Can you work these out from the model? Positions are in its coordinate system, mm. Coordinates: 2 decimals unless noted, no trailing zeros. Order: outer loops, then holes, each group sorted by start corner. A loop starts at its lowest first (then second) coordinate and runs counter-clockwise, first axis right, second up. Notation, with made-up numbers: (31, 31) -> (47, 31) arc R29 cw to (47, 61) -> close; hole circle Ø1 at (31, 22). An arc over 180 degrees is marked (long way). Answer as a JSON object with one key per item and string values. Group by question number.
(1) I want a section at D-D, the plane y = -48. List the corners of the cut face in (x, z) for me, plus the area to 3 significant figures.
(2) For pin 1 (2 mm diameter, centred on y = 36.5, z = 1.5, fed in from +X); pin 2 (1.5 mm diameter, centred on x = 283.5, z = 1, fed in from +Y); pin 3 (2 mm diameter, centred on x = 274, z = 3, fed in from +Y), each with a flat end and sliding along its axis, tell me the tip position at first contact or that it passes through.
(3) I want a section at A-A, the plane x = 285.5. List the corners of the cut face in (y, z) for me, plus the area to 3 significant figures.
(4) I want a section at B-B, the plane z = 0.8. List the corners of the cut face in (x, y) for me, plus the area to 3 significant figures.
(5) I need wall thicknesses on line 1 (Y direction, x = 282, z = 2.65); line 2 (Y direction, x = 284, z = 2.4); line 3 (X direction, y = 17, z = 2.6). Which ranges of each line are inside material? Lowest first, please.
(6) I want a section at C-C, the plane x = 279.5. List the corners of the cut face in (y, z) for me, plus the area to 3 significant figures.
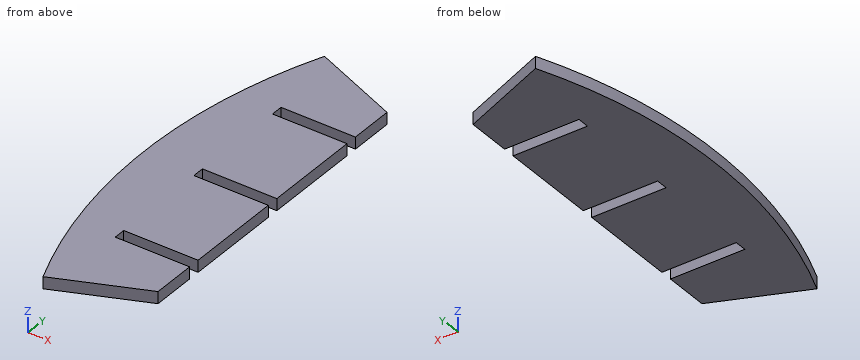
Autodesk Inventor part; units mm, degrees
ref_plane "Work Plane1" through (0, 0, 0) normal (0, 0, 1) x (1, 0, 0)
ref_plane "YZ Plane" through (0, 0, 0) normal (1, 0, 0) x (0, 1, 0)
ref_plane "XZ Plane" through (0, 0, 0) normal (0, 1, 0) x (-1, 0, 0)
ref_plane "Work Plane1" through (0, 0, 0) normal (0, 0, 1) x (1, 0, 0)
sketch "Sketch1" plane through (0, 0, 0) normal (0, 0, 1) x (1, 0, 0)
  line L0 (300, 300) -> (-300, 300) construction
  line L1 (-300, 300) -> (-300, -300) construction
  line L2 (-300, -300) -> (300, -300) construction
  line L3 (300, -300) -> (300, 300) construction
  line L4 (300, -53.8478) -> (-254.3277, -283.4578) construction
  arc A0 (269.6349, -64.9002) -> (269.6349, -64.9002) centre (430, 0) ccw construction
  arc A1 (269.2287, 63.8872) -> (269.6349, -64.9002) centre (430, 0) ccw construction
  arc A2 (269.2287, 63.8872) -> (269.2287, 63.8872) centre (430, 0) ccw construction
  line L5 (-254.3277, 283.4578) -> (300, 53.8478) construction
  line L6 (300, 53.8478) -> (300, -53.8478)
  line L7 (270.1688, -66.2042) -> (300, -53.8478)
  line L8 (270.1688, 66.2042) -> (300, 53.8478)
  arc A3 (270.1688, 66.2042) -> (270.1688, -66.2042) centre (430, 0) ccw
  line L9 (300, -35) -> (275, -35)
  line L10 (275, -35) -> (275, -39)
  line L11 (275, -39) -> (300, -39)
  line L12 (300, -39) -> (300, -35)
  line L13 (300, 2) -> (275, 2)
  line L14 (275, 2) -> (275, -2)
  line L15 (275, -2) -> (300, -2)
  line L16 (300, -2) -> (300, 2)
  line L17 (300, 39) -> (275, 39)
  line L18 (275, 39) -> (275, 35)
  line L19 (275, 35) -> (300, 35)
  line L20 (300, 35) -> (300, 39)
  point P0 (0, 0)
  point P1 (300, 0)
  dimension "d2" = 25
  dimension "d3" = 4
  dimension "d4" = 25
  dimension "d5" = 4
  dimension "d6" = 25
  dimension "d7" = 4
  dimension "d8" = 35
  dimension "d9" = 35
extrude "Extrusion2" add sketch "Sketch1" along normal blind 4 contours L6 L17 L18 L19 L13 L14 L15 L9 L10 L11 L7 A3 L8
equation "\"d3\" = d7"
equation "\"d5\" = d7"
properties part number "frontformer" material "Wood (Cherry)"
Computed values:
{
 "1": {"outline": "(263.79, 0) -> (300, 0) -> (300, 4) -> (263.79, 4) -> close", "area": "145 mm2"},
 "2": {"pin 1": "stops at x = 275", "pin 2": "stops at y = 60.99", "pin 3": "stops at y = 65.03"},
 "3": {"outline": "(-59.85, 0) -> (-39, 0) -> (-39, 4) -> (-59.85, 4) -> close; (-35, 0) -> (-2, 0) -> (-2, 4) -> (-35, 4) -> close; (2, 0) -> (35, 0) -> (35, 4) -> (2, 4) -> close; (39, 0) -> (59.85, 0) -> (59.85, 4) -> (39, 4) -> close", "area": "431 mm2"},
 "4": {"outline": "(270.17, -66.2) -> (300, -53.85) -> (300, -39) -> (275, -39) -> (275, -35) -> (300, -35) -> (300, -2) -> (275, -2) -> (275, 2) -> (300, 2) -> (300, 35) -> (275, 35) -> (275, 39) -> (300, 39) -> (300, 53.85) -> (270.17, 66.2) arc R173 ccw to start", "area": "4,450 mm2"},
 "5": {"line 1": "y = -61.3 to -39, -35 to -2, 2 to 35, 39 to 61.3", "line 2": "y = -60.48 to -39, -35 to -2, 2 to 35, 39 to 60.48", "line 3": "x = 257.84 to 300"},
 "6": {"outline": "(-62.34, 0) -> (-39, 0) -> (-39, 4) -> (-62.34, 4) -> close; (-35, 0) -> (-2, 0) -> (-2, 4) -> (-35, 4) -> close; (2, 0) -> (35, 0) -> (35, 4) -> (2, 4) -> close; (39, 0) -> (62.34, 0) -> (62.34, 4) -> (39, 4) -> close", "area": "451 mm2"}
}
